from build123d import *

# Parameters (mm, degrees)
F0_W           = 152.4
F0_H           = 152.4
F1_DEPTH       = 63.5
F3_DEPTH       = 63.17996
F4_DEPTH       = 12.7
F6_DEPTH       = 609.6
F7_W           = 152.4
F7_H           = 56.7961266285
F8_DEPTH       = 0.16002
F8_DEPTH_BACK  = 0.16002
F9_W           = 152.4
F9_H           = 56.7961266285
F10_DEPTH      = 0.16002
F10_DEPTH_BACK = 0.16002
F12_DEPTH      = 0.32004
F19_DEPTH      = 127
F24_D          = 9.525
F24_DEPTH      = 38.1
F24_TIP        = 2.8615986981
F26_DEPTH      = 25.4


with BuildPart() as f1:
    # F0 (on Top) → F1 (new body)
    with BuildSketch(Plane.XY):
        with Locations((22.6197618335, 8.0124375336)):
            Rectangle(F0_W, F0_H)
    extrude(amount=F1_DEPTH)

    # F2 (on face) → F3 (cut)
    with BuildSketch(Plane.XY.offset(63.5)):
        Polygon((22.6197618335, 83.8923975336), (-53.2601981665, 83.8923975336), (-53.2601981665, -0.1986662101), (-53.2601981665, -67.8672684664), (22.6197618335, -67.8672684664), (98.4997218335, -67.8672684664), (98.4997218335, -5.9687194955), (98.4997218335, 83.8923975336), align=None)
    extrude(amount=-F3_DEPTH, mode=Mode.SUBTRACT)

    # F4 (cut): a face of the model
    f4_faces = [f1.faces().sort_by_distance(p)[0] for p in [
        (22.6197618335, 83.9969113867, 63.5),
    ]]
    extrude(f4_faces, amount=-F4_DEPTH, mode=Mode.SUBTRACT)

    # F5 (on face) → F6 (cut)
    with BuildSketch(Plane(origin=(0, 84.2124375336, 0), x_dir=(-1, 0, 0), z_dir=(0, 1, 0))):
        Polygon((-73.4197618335, 0), (-98.8197618335, 50.8), (-98.8197618335, 0), align=None)
        Polygon((53.5802381665, 0), (53.5802381665, 50.8), (28.1802381665, 0), align=None)
    extrude(amount=-F6_DEPTH, mode=Mode.SUBTRACT)

    # F7 (on face) → F8 (join, two sides)
    with BuildSketch(Plane(origin=(58.7358094668, 0, -29.3679047334), x_dir=(0, 1, 0), z_dir=(0.894427191, 0, -0.4472135955))) as f8_sk:
        with Locations((8.0124375336, 61.2323789846)):
            Rectangle(F7_W, F7_H)
    extrude(amount=-F8_DEPTH)
    extrude(f8_sk.sketch, amount=F8_DEPTH_BACK)

    # F9 (on face) → F10 (join, two sides)
    with BuildSketch(Plane(origin=(-22.5441905332, 0, -11.2720952666), x_dir=(0, -1, 0), z_dir=(-0.894427191, 0, -0.4472135955))) as f10_sk:
        with Locations((-8.0124375336, 41.0006489467)):
            Rectangle(F9_W, F9_H)
    extrude(amount=F10_DEPTH)
    extrude(f10_sk.sketch, amount=-F10_DEPTH_BACK)

    # F11 (on face) → F12 (join)
    with BuildSketch(Plane.XY.offset(0.32004)):
        Polygon((73.4008740347, -67.8672684664), (-28.1613503676, -67.8672684664), (22.6197618335, -118.6483806675), align=None)
    extrude(amount=F12_DEPTH)

    # F13 (on face) → F14 section 0
    with BuildSketch(Plane.XY.offset(50.8)):
        Polygon((98.6408540347, -68.1875624664), (-53.4013303676, -68.1875624664), (22.6690676063, -118.3943599463), align=None)
    # F12_face (on face) → F14 section 1
    with BuildSketch(Plane(origin=(22.6197618335, -85.0078352001, 0.64008), x_dir=(1, 0, 0), z_dir=(0, 0, 1))):
        Polygon((-50.4608182011, 16.8202727337), (0, -33.6405454674), (50.4608182011, 16.8202727337), align=None)
    loft()

    # F18 (on face) → F19 (join)
    with BuildSketch(Plane(origin=(0, 84.2124375336, 0), x_dir=(-1, 0, 0), z_dir=(0, 1, 0))):
        with BuildLine():
            Line((53.4371119273, 50.8715631196), (53.7233644056, 50.7284368804))
            ThreePointArc((53.7233644056, 50.7284368804), (-22.4229632548, 126.9463276603), (-98.6408540347, 50.8))
            Line((-98.6408540347, 50.8), (-98.3208140347, 50.8))
            ThreePointArc((-98.3208140347, 50.8), (-22.464787963, 126.6661203454), (53.4114253128, 50.8201898905))
            Line((53.4114253128, 50.8201898905), (53.4371119273, 50.8715631196))
        make_face()
    extrude(amount=-F19_DEPTH)

    # F15 (on face) → F20 section 0
    with BuildSketch(Plane.XY.offset(50.8)):
        Polygon((-49.3224896491, -67.8672684664), (22.6690676063, -113.2092401385), (95.3528803221, -67.8672684664), align=None)
    # F17 (on offset) → F20 section 1
    with BuildSketch(Plane(origin=(0, 0, 2.54), x_dir=(1, 0, 0), z_dir=(0, 0, -1))):
        Polygon((23.141015321, 113.2561042905), (-28.1210406962, 67.4263015389), (71.8552097678, 67.4263015389), align=None)
    loft(mode=Mode.SUBTRACT)

    # F24
    with Locations(Plane(origin=(0, 84.2124375336, 0), x_dir=(-1, 0, 0), z_dir=(0, 1, 0))):
        with Locations((-36.7363579571, 12.5697767362)):
            Hole(F24_D / 2, depth=F24_DEPTH)
            with Locations((0, 0, -(F24_DEPTH + F24_TIP / 2))):  # 118° drill point
                Cone(0, F24_D / 2, F24_TIP, mode=Mode.SUBTRACT)

    # F25 (on face) → F26 (cut)
    with BuildSketch(Plane(origin=(0, 84.2124375336, 0), x_dir=(-1, 0, 0), z_dir=(0, 1, 0))):
        with BuildLine():
            ThreePointArc((-16.1407376707, 12.6165375113), (-11.3782376707, 7.8540375113), (-6.6157376707, 12.6165375113))
            ThreePointArc((-6.6157376707, 12.6165375113), (-11.3782376707, 17.3790375113), (-16.1407376707, 12.6165375113))
        make_face()
    extrude(amount=-F26_DEPTH, mode=Mode.SUBTRACT)


solid = f1.part
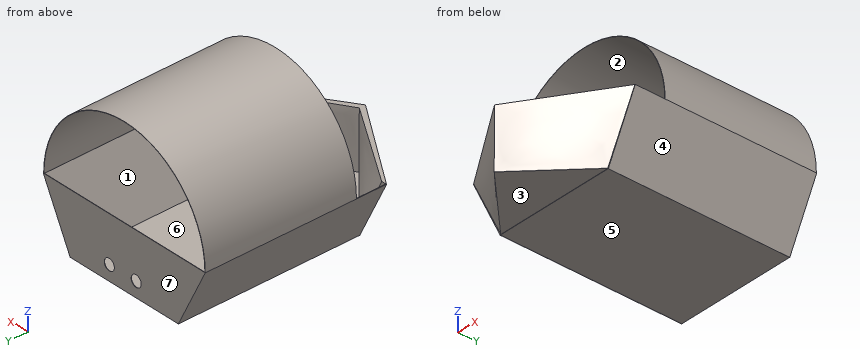
Can you work these out from the model? Positions are in its coordinate system, mm. Face numbers are marked on the shaded views. A direction names the side the tool comes from. Give positions to 0.01 mm unless a question says otherwise; leave off trailing zeros. Loops run counter-clockwise (first coordinate to the right, second up) from the corner with the lowest first, then second, coordinate; pieces in that order, holes last. Notation, with made-up numbers: M 34.25,67.5 L 51.25,67.5 A18 ccw 51.25,99.5 Z; hole C 48.25,55.25 d3. An arc over 180 degrees is marked long. One line per item, written item: value.
1) Imagine slicing it at D-D on x = 9.5. Count the separate pieces of the cut face and the enclosed holes in it, and give its area (3 significant figures).
Geometry check:
separate pieces: 3
enclosed holes: 0
area: 414 mm²
2) On a 3-axis mill with a long thin cutter (end or side, diameter ignored), from which of +Z, -Z, +X, -X, +Y, -Y can I reach the whole of each face in a straight line? I mean the marked faces 1, 2, 3 and 4. Say none if no direction works.
Geometry check:
face 1: none
face 2: +Y, -Y
face 3: -Z, +X, -X, -Y
face 4: -Z, +X, +Y, -Y
3) Imagine slicing it at C-C on z = 74. Write out the boundary of the cut face in (x, y).
Geometry check:
outline: M -50.09,-42.79 L -49.78,-42.79 L -49.78,84.21 L -50.09,84.21 Z; M 94.69,-42.79 L 95.01,-42.79 L 95.01,84.21 L 94.69,84.21 Z
4) I'm going to push flat-ended pins straight in: pin 1 (10 mm diameter, centred on y = -10.5, z = 109.5, fed in from -X); pin 2 (15 mm diameter, centred on x = 33, y = -86, fed in from -Z); pin 3 (1 mm diameter, centred on x = 37.5, z = 13.5, fed in from +Y). Where does each tip first touch, or does it pass through?
Geometry check:
pin 1: stops at x = -31.54
pin 2: stops at z = 0.32
pin 3: stops at y = -100.61
5) Thinking about a two-plate mould opening in Y: for the marked faces 5, 6 and 7, which applies, +Y half, -Y half, draft (parallel to the pull), parting line (faces both ways), or undercut?
Geometry check:
face 5: draft
face 6: undercut
face 7: +Y half
6) Please list where these lines run through material, in increasing order: line 1 (Z direction, x = 32, y = 72.5); line 2 (Z direction, x = -16.5, y = 71.5); line 3 (X direction, y = -12.5, z = 33).
Geometry check:
line 1: z = 0 to 0.32, 126.06 to 126.35
line 2: z = 0 to 0.32, 115.9 to 116.23
line 3: x = -44.86 to -44.5, 89.74 to 90.1
7) Imagine slicing it at A-A on z = 117. Write out the boundary of the cut face in (x, y).
Geometry check:
outline: M -15.18,-42.79 L -14.6,-42.79 L -14.6,84.21 L -15.18,84.21 Z; M 59.51,-42.79 L 60.1,-42.79 L 60.1,84.21 L 59.51,84.21 Z
